Autodesk Inventor part; units mm, degrees
ref_plane "YZ Plane" through (0, 0, 0) normal (1, 0, 0) x (0, 1, 0)
ref_plane "XZ Plane" through (0, 0, 0) normal (0, 1, 0) x (-1, 0, 0)
ref_plane "XY Plane" through (0, 0, 0) normal (0, 0, 1) x (1, 0, 0)
sketch "Sketch1" plane through (0, 0, 0) normal (0, 0, 1) x (1, 0, 0)
  line L0 (-8.5, 48.5) -> (8.5, 48.5)
  line L1 (48.5, 8.5) -> (48.5, -8.5)
  line L2 (8.5, -48.5) -> (-8.5, -48.5)
  line L3 (-48.5, -8.5) -> (-48.5, 8.5)
  circle A0 centre (0, 0) radius 41.25
  circle A1 centre (0, 0) radius 8.45
  circle A2 centre (0, 0) radius 4
  arc A3 (48.5, 8.5) -> (8.5, 48.5) centre (8.5, 8.5) ccw
  arc A4 (8.5, -48.5) -> (48.5, -8.5) centre (8.5, -8.5) ccw
  arc A5 (-48.5, -8.5) -> (-8.5, -48.5) centre (-8.5, -8.5) ccw
  arc A6 (-8.5, 48.5) -> (-48.5, 8.5) centre (-8.5, 8.5) ccw
  point P0 (-48.5, 48.5)
  point P1 (48.5, -48.5)
  point P2 (48.5, 48.5)
  point P3 (-48.5, -48.5)
  point P4 (0, 48.5)
  point P5 (48.5, 0)
  dimension "d0" = 97
  dimension "d1" = 82.5
  dimension "d2" = 16.9
  dimension "d3" = 8
  dimension "d10" = 40
extrude "Extrusion1" add sketch "Sketch1" along normal blind 2 contours A1
extrude "Extrusion2" add sketch "Sketch1" along normal blind 7 contours A0
extrude "Extrusion3" add sketch "Sketch1" along normal blind 18 contours L0 A3 L1 A4 L2 A5 L3 A6
sketch "Sketch3" plane through (0, 0, 18) normal (0, 0, 1) x (1, 0, 0)
  circle A0 centre (0, 0) radius 41.25
  line L0 (21.9501, 34.925) -> (64.9501, 34.925)
  line L1 (41.9501, 40.25) -> (47.9501, 40.25)
  line L2 (49.9501, 42.25) -> (64.9501, 42.25)
  line L3 (40.9501, 41.25) -> (28.9501, 41.25)
  line L4 (49.9501, 42.25) -> (47.9501, 40.25)
  line L5 (40.9501, 41.25) -> (41.9501, 40.25)
  line L6 (47.9501, 40.25) -> (64.9501, 40.25) construction
  line L7 (41.9501, 40.25) -> (28.9501, 40.25) construction
  line L8 (64.9501, 42.25) -> (64.9501, 34.925)
  line L9 (28.9501, 37.925) -> (21.9501, 37.925)
  line L10 (28.9501, 37.925) -> (28.9501, 41.25)
  line L11 (21.9501, 37.925) -> (21.9501, 34.925) construction
  line L12 (21.9501, 34.925) -> (16.225193, 34.925)
  line L13 (21.9501, 37.925) -> (16.225193, 37.925)
  line L14 (16.225193, 34.925) -> (16.225193, 37.925)
  circle A1 centre (0, 0) radius 4
  line L15 (0, 0) -> (48.5, 0)
  line L16 (48.5, -8.5) -> (48.5, 8.5)
  line L17 (21.9501, -34.925) -> (64.9501, -34.925)
  line L18 (41.9501, -40.25) -> (47.9501, -40.25)
  line L19 (49.9501, -42.25) -> (64.9501, -42.25)
  line L20 (40.9501, -41.25) -> (28.9501, -41.25)
  line L21 (49.9501, -42.25) -> (47.9501, -40.25)
  line L22 (40.9501, -41.25) -> (41.9501, -40.25)
  line L23 (47.9501, -40.25) -> (64.9501, -40.25) construction
  line L24 (41.9501, -40.25) -> (28.9501, -40.25) construction
  line L25 (64.9501, -42.25) -> (64.9501, -34.925)
  line L26 (28.9501, -37.925) -> (21.9501, -37.925)
  line L27 (28.9501, -37.925) -> (28.9501, -41.25)
  line L28 (21.9501, -37.925) -> (21.9501, -34.925) construction
  line L29 (21.9501, -34.925) -> (16.225193, -34.925)
  line L30 (21.9501, -37.925) -> (16.225193, -37.925)
  line L31 (16.225193, -34.925) -> (16.225193, -37.925)
  line L32 (28.9501, -37.925) -> (64.9501, -37.925)
  point P0 (16.225193, -37.925)
  dimension "d12" = 10.65
  dimension "d13" = 14.65
  dimension "d14" = 12.65
  dimension "d15" = 45
  dimension "d16" = 45
  dimension "d17" = 15
  dimension "d18" = 6
  dimension "d19" = 12
  dimension "d21" = 7
  dimension "d22" = 6
sketch "Sketch3 outline for Revolution1" plane through (0, 0, 18) normal (0, 0, 1) x (1, 0, 0)
  line L0 (64.9501, 34.925) -> (64.9501, 42.25)
  line L1 (21.9501, 34.925) -> (64.9501, 34.925)
  arc A0 (16.225193, 37.925) -> (21.9501, 34.925) centre (0, 0) cw
  line L2 (21.9501, 37.925) -> (16.225193, 37.925)
  line L3 (28.9501, 37.925) -> (21.9501, 37.925)
  line L4 (28.9501, 41.25) -> (28.9501, 37.925)
  line L5 (40.9501, 41.25) -> (28.9501, 41.25)
  line L6 (41.9501, 40.25) -> (40.9501, 41.25)
  line L7 (47.9501, 40.25) -> (41.9501, 40.25)
  line L8 (49.9501, 42.25) -> (47.9501, 40.25)
  line L9 (64.9501, 42.25) -> (49.9501, 42.25)
revolve "Revolution1" cut sketch "Sketch3 outline for Revolution1" angle 360 about axis through (21.9501, 34.925, 18) along (1, 0, 0)
sketch "Sketch3 outline for Revolution2" plane through (0, 0, 18) normal (0, 0, 1) x (1, 0, 0)
  line L0 (21.9501, -37.925) -> (28.9501, -37.925)
  line L1 (16.225193, -37.925) -> (21.9501, -37.925)
  arc A0 (21.9501, -34.925) -> (16.225193, -37.925) centre (0, 0) cw
  line L2 (64.9501, -34.925) -> (21.9501, -34.925)
  line L3 (64.9501, -37.925) -> (64.9501, -34.925)
  line L4 (28.9501, -37.925) -> (64.9501, -37.925)
revolve "Revolution2" cut sketch "Sketch3 outline for Revolution2" angle 360 about axis through (21.9501, -34.925, 18) along (1, 0, 0)
sketch "Sketch4" plane through (0, 0, 18) normal (0, 0, 1) x (1, 0, 0)
  line L0 (35.59556, -37.925) -> (16.225193, -37.925) construction
  arc A0 (16.225193, 37.925) -> (16.225193, -37.925) centre (0, 0) ccw construction
  line L1 (16.225193, 37.925) -> (28.9501, 37.925) construction
  line L2 (28.9501, 37.925) -> (28.9501, 41.25) construction
  line L3 (28.9501, 41.25) -> (31.466007, 41.25) construction
  arc A1 (31.466007, 41.25) -> (8.5, 48.5) centre (8.5, 8.5) ccw construction
  line L4 (8.5, 48.5) -> (-8.5, 48.5) construction
  arc A2 (-8.5, 48.5) -> (-48.5, 8.5) centre (-8.5, 8.5) ccw construction
  line L5 (-48.5, 8.5) -> (-48.5, -8.5) construction
  arc A3 (-48.5, -8.5) -> (-8.5, -48.5) centre (-8.5, -8.5) ccw construction
  line L6 (-8.5, -48.5) -> (8.5, -48.5) construction
  arc A4 (8.5, -48.5) -> (35.59556, -37.925) centre (8.5, -8.5) ccw construction
  line L7 (26.121962, -31.925) -> (40.923284, -31.925) construction
  arc A5 (40.923284, -31.925) -> (48.5, -8.5) centre (8.5, -8.5) ccw construction
  line L8 (48.5, -8.5) -> (48.5, 8.5) construction
  arc A6 (48.5, 8.5) -> (42.482201, 29.6) centre (8.5, 8.5) ccw construction
  line L9 (42.482201, 29.6) -> (41.9501, 29.6) construction
  line L10 (41.9501, 29.6) -> (40.9501, 28.6) construction
  line L11 (40.9501, 28.6) -> (29.725452, 28.6) construction
  arc A7 (26.121962, -31.925) -> (29.725452, 28.6) centre (0, 0) ccw construction
  line L12 (-48.5, 0) -> (-41.25, 0) construction
  circle A8 centre (-44.875, 0) radius 1.485
  circle A9 centre (0, -44.875) radius 1.485
  circle A10 centre (44.875, 0) radius 1.485
  circle A11 centre (0, 44.875) radius 1.485
  dimension "d25" = 2.97
  dimension "d28" = 360
extrude "Extrusion4" cut sketch "Sketch4" against normal through all
properties part number "Case"
The model under review builds one solid part; all positions refer to its coordinate system, in mm. A direction names the side the tool comes from. Round coordinates to 2 decimals unless told otherwise and drop trailing zeros. Order: outer loops, then holes, each group sorted by start corner. A loop starts at its lowest first (then second) coordinate and runs counter-clockwise, first axis right, second up.
Item 1: Machinability: for faces 5 (the flat face through (-1, -9, 7)), 6 (the cylindrical face through (23.9, 36, 15.2)), 7 (the flat face through (-48.5, 0, 9)), 8 (the conical face through (41.443, 29.608, 15.603)), 9 (the cylindrical face through (-36.472, -37.094, 8.874)), which of the approach directions +Z, -Z, +X, -X, +Y, -Y give a long, thin tool a straight path to every point of the face, cutting with its end or side? Answer none if there is none.
Working result:
face 5: +Z
face 6: +Z, +X
face 7: +Z, -Z, -X, +Y, -Y
face 8: +Z, +Y
face 9: +Z, -Z, -X, -Y
Item 2: Add section D-D, the plane y = 18. State the section outline as (x, z) points, and give its area (3 significant figures).
Working result:
outline: (-47.36, 0) - (47.36, 0) - (47.36, 18) - (37.12, 18) - (37.12, 7) - (-37.12, 7) - (-37.12, 18) - (-47.36, 18) - close
area: 888 mm2
Item 3: Draft analysis for pull direction X (two halves, no side actions). For faces 1 (the cylindrical face through (0.798, -43.623, 9.126)), 2 (the cylindrical face through (33.53, 32.89, 12.01)), 3 (the cylindrical face through (36.472, 37.094, 8.874)), 4 (the flat face through (0, 48.5, 9)), state which applies: released by +X, released by -X, zero draft, split by the parting line, or undercut.
Working result:
face 1: undercut
face 2: undercut
face 3: released by +X
face 4: zero draft
Item 4: Add section A-A, the plane y = 0. State the section outline as (x, z) points.
Working result:
outline: (-48.5, 0) - (-46.36, 0) - (-46.36, 18) - (-48.5, 18) - close; (-43.39, 0) - (-4, 0) - (-4, 2) - (-8.45, 2) - (-8.45, 7) - (-41.25, 7) - (-41.25, 18) - (-43.39, 18) - close; (4, 0) - (43.39, 0) - (43.39, 18) - (41.25, 18) - (41.25, 7) - (8.45, 7) - (8.45, 2) - (4, 2) - close; (46.36, 0) - (48.5, 0) - (48.5, 18) - (46.36, 18) - close
Item 5: For pin 1 (5 mm diameter, centred on x = 0, y = 44.875, fed in from -Z); pin 2 (8 mm diameter, centred on x = 27, z = 5.5, fed in from +Y); pin 3 (10 mm diameter, centred on x = -31, z = 6.5, fed in from -Y); pin 4 (6 mm diameter, centred on x = 17, z = 12, fed in from -Y), all flat-tipped, find the tip position at first contact; note any pin that passes through.
Working result:
pin 1: stops at z = 0
pin 2: stops at y = 45.78
pin 3: stops at y = -44.47
pin 4: stops at y = -48.12
Item 6: To check wall thickness, follow probe 1 along Y at (x, z) = (0, 3.4); probe 2 along Y at (x, z) = (0, 16); probe 3 along Z at (x, y) = (-15.5, 38). State the ranges of each line that lie inside material, in increasing order.
Working result:
probe 1: y = -48.5 to -46.36, -43.39 to -8.45, 8.45 to 43.39, 46.36 to 48.5
probe 2: y = -48.5 to -46.36, -43.39 to -41.25, 41.25 to 43.39, 46.36 to 48.5
probe 3: z = 0 to 7
Item 7: Add section C-C, the plane z = 4. State the section outline as (x, y) points (3 decimals), and give its area (3 significant figures).
Working result:
outline: (-48.5, -8.5) arc R40 ccw to (-8.5, -48.5) - (8.5, -48.5) arc R40 ccw to (48.5, -8.5) - (48.5, 8.5) arc R40 ccw to (8.5, 48.5) - (-8.5, 48.5) arc R40 ccw to (-48.5, 8.5) - close; hole circle Ø2.97 at (-44.875, 0); hole circle Ø16.9 at (0, 0); hole circle Ø2.97 at (0, -44.875); hole circle Ø2.97 at (0, 44.875); hole circle Ø2.97 at (44.875, 0)
area: 7,780 mm2
